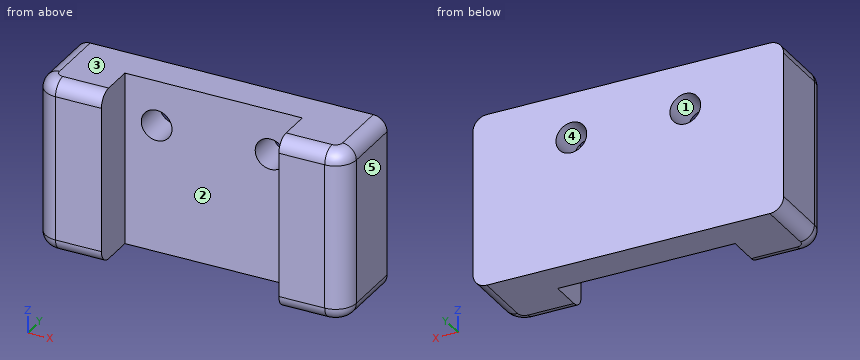
```python
from build123d import *

# Parameters (mm, degrees)
BOSS_EXTRUDE1_DEPTH = 25
SKETCH2_R           = 2.225
CUT_EXTRUDE1_DEPTH  = 36.545745174
FILLET1_R           = 3
FILLET2_R           = 2


with BuildPart() as part:
    # Sketch1 → Boss-Extrude1 (new body)
    with BuildSketch(Plane.XY):
        Polygon((-22.5, 5), (22.5, 5), (22.5, -6.5), (12.85, -6.5), (12.85, 0), (-12.85, 0), (-12.85, -6.5), (-22.5, -6.5), align=None)
    extrude(amount=BOSS_EXTRUDE1_DEPTH)

    # Sketch2 → Cut-Extrude1 (cut, through all)
    with BuildSketch(Plane(origin=(0, 5, 0), x_dir=(1, 0, 0), z_dir=(0, 1, 0))):
        with Locations(Location((-8.25, -18.5, 0), (0, 0, 270))):
            Circle(SKETCH2_R)
        with Locations(Location((8.25, -18.5, 0), (0, 0, 270))):
            Circle(SKETCH2_R)
    extrude(amount=-CUT_EXTRUDE1_DEPTH, mode=Mode.SUBTRACT)

    # Fillet1
    fillet1_edges = [part.edges().sort_by_distance(p)[0] for p in [
        (22.5, -6.5, 12.5),
        (-22.5, -6.5, 12.5),
    ]]
    fillet(fillet1_edges, radius=FILLET1_R)

    # Fillet2
    fillet2_edges = [part.edges().sort_by_distance(p)[0] for p in [
        (-22.5, 0.75, 0),
        (16.175, -6.5, 25),
        (22.5, 0.75, 0),
        (22.5, 0.75, 25),
        (-16.175, -6.5, 0),
        (-21.621320344, -5.621320344, 0),
        (21.621320344, -5.621320344, 0),
        (-16.175, -6.5, 25),
        (-21.621320344, -5.621320344, 25),
        (21.621320344, -5.621320344, 25),
        (-22.5, 0.75, 25),
        (16.175, -6.5, 0),
    ]]
    fillet(fillet2_edges, radius=FILLET2_R)


solid = part.part
```
Read the model definition and answer for the solid it produces. Units are mm, in the model's axes. Face numbers are marked on the shaded views. A direction names the side the tool comes from. Give positions to 0.01 mm unless a question says otherwise; leave off trailing zeros. Order: outer loops, then holes, each group sorted by start corner. A loop starts at its lowest first (then second) coordinate and runs counter-clockwise, first axis right, second up. Notation, with made-up numbers: (76.5, 52) -> (125.5, 52) arc R29 ccw to (125.5, 82) -> close; hole circle Ø10 at (12.5, -35.75). An arc over 180 degrees is marked (long way). One line per item, written item: value. Start each with the question number.
(1) The part is cut by section B-B (z = 18.5). Determine the outline of the cut face in (x, y) (3 decimals).
(2) For a pull along X with two mould halves and no side action, classify the marked faces 3, 4 and 5 as released by +X, released by -X, zero draft, split by the parting line, or undercut.
(3) The part is cut by section C-C (y = -2.25). Determine the outline of the cut face in (x, z).
(4) The part is cut by section D-D (z = 12.75). Determine the outline of the cut face in (x, y), and give its area (3 significant figures).
(5) Flat-ended cylindrical pins translate along their axes: P1, Ø8, axis at x = -0.5, z = 8, coming from the -Y side; P2, Ø6, axis at x = 8.25, z = 18.5, coming from the +Y side. Find the tip coordinate at first contact, or state that the pin passes through.
(6) The part is cut by section A-A (x = -8.25). Determine the outline of the cut face in (y, z) (3 decimals), and give its area (3 significant figures).
(7) A tool of negligible diameter and unlimited length cuts with its end or side. For the marked faces 1 and 2, from which of +Z, -Z, +X, -X, +Y, -Y can it reach the whole face along a straight path? Write none if from no direction.
(8) Straight lines are drawn through the part: L1, parallel to X at y = 3.25, z = 18.5 (3 decimals); L2, parallel to X at y = -1.75, z = 15.5; L3, parallel to X at y = 3, z = 17. For each, find the intervals that lie inside material, in ascending order.
Taken from the geometry:
1. outline: (-22.5, -3.5) arc R3 ccw to (-19.5, -6.5) -> (-12.85, -6.5) -> (-12.85, 0) -> (-10.475, 0) -> (-10.475, 5) -> (-22.5, 5) -> close; (-6.025, 0) -> (6.025, 0) -> (6.025, 5) -> (-6.025, 5) -> close; (10.475, 0) -> (12.85, 0) -> (12.85, -6.5) -> (19.5, -6.5) arc R3 ccw to (22.5, -3.5) -> (22.5, 5) -> (10.475, 5) -> close
2. face 3: zero draft
2. face 4: undercut
2. face 5: released by +X
3. outline: (-22.5, 2) arc R2 ccw to (-20.5, 0) -> (-12.85, 0) -> (-12.85, 25) -> (-20.5, 25) arc R2 ccw to (-22.5, 23) -> close; (12.85, 0) -> (20.5, 0) arc R2 ccw to (22.5, 2) -> (22.5, 23) arc R2 ccw to (20.5, 25) -> (12.85, 25) -> close
4. outline: (-22.5, -3.5) arc R3 ccw to (-19.5, -6.5) -> (-12.85, -6.5) -> (-12.85, 0) -> (12.85, 0) -> (12.85, -6.5) -> (19.5, -6.5) arc R3 ccw to (22.5, -3.5) -> (22.5, 5) -> (-22.5, 5) -> close
4. area: 347 mm^2
5. P1: y = 0
5. P2: y = 5
6. outline: (0, 0) -> (5, 0) -> (5, 16.275) -> (0, 16.275) -> close; (0, 20.725) -> (5, 20.725) -> (5, 25) -> (0, 25) -> close
6. area: 103 mm^2
7. face 1: +Y, -Y
7. face 2: +Z, -Z, -Y
8. L1: -22.5 to -10.475, -6.025 to 6.025, 10.475 to 22.5
8. L2: -22.5 to -12.85, 12.85 to 22.5
8. L3: -22.5 to -9.89, -6.61 to 6.61, 9.89 to 22.5
